```python
from build123d import *

# Parameters (mm, degrees)
BOSS_EXTRUDE1_DEPTH = 20
FILLET1_R           = 1
FILLET2_R           = 0.5


with BuildPart() as part:
    # Sketch1 → Boss-Extrude1 (new body)
    with BuildSketch(Plane(origin=(0, 0, 0), x_dir=(1, 0, 0), z_dir=(0, 1, 0))):
        Polygon((-2.4, 4.581818182), (2.4, 4.581818182), (7, 0.381818182), (2.4, 0.381818182), (2.4, -1.618181818), (10, -1.618181818), (10, -4.618181818), (-10, -4.618181818), (-10, -1.618181818), (-2.4, -1.618181818), (-2.4, 0.381818182), (-7, 0.381818182), align=None)
    extrude(amount=BOSS_EXTRUDE1_DEPTH)

    # Fillet1
    fillet1_edges = [part.edges().sort_by_distance(p)[0] for p in [
        (7, 10, -0.381818182),
        (-7, 10, -0.381818182),
        (-2.4, 10, -4.581818182),
        (2.4, 10, -4.581818182),
    ]]
    fillet(fillet1_edges, radius=FILLET1_R)

    # Fillet2
    fillet2_edges = [part.edges().sort_by_distance(p)[0] for p in [
        (2.4, 10, -0.381818182),
        (2.4, 10, 1.618181818),
        (-2.4, 10, 1.618181818),
        (-2.4, 10, -0.381818182),
    ]]
    fillet(fillet2_edges, radius=FILLET2_R)


solid = part.part
```
Here's how the part is built. I have some questions about the finished solid (model axes, mm). A direction names the side the tool comes from. Coordinates: 2 decimals unless noted, no trailing zeros. Order: outer loops, then holes, each group sorted by start corner. A loop starts at its lowest first (then second) coordinate and runs counter-clockwise, first axis right, second up. Notation, with made-up numbers: (2, 9) - (58, 9) arc R10 ccw to (58, 23) - close; hole circle Ø11 at (-18.5, -28.5). An arc over 180 degrees is marked (long way). One line per question, with ' | ' between items. Start each with the question number.
1. Please list where these lines run through material, in increasing order: line 1 along Z through (x, y) = (-4.25, 17.25); line 2 along Z through (x, y) = (4.5, 12.75); line 3 along Z through (x, y) = (-7, 19.25). Write a range as [from, to].
2. If we section it at C-C (x = 8): Write out the boundary of the cut face in (y, z), and give its area (3 significant figures).
3. If we section it at D-D (z = 0.75): Write out the boundary of the cut face in (x, y), and give its area (3 significant figures).
4. If we section it at A-A (y = 6.75): Write out the boundary of the cut face in (x, z).
5. I'm going to push flat-ended pins straight in: pin 1 Ø2 at (x, y) = (6, 12.5) entering from -Z; pin 2 Ø3.5 at (x, y) = (-7, 12.5) entering from -Z; pin 3 Ø1.5 at (x, y) = (-4, 13.5) entering from -Z; pin 4 Ø4 at (x, y) = (3.5, 2) entering from -Z. Where does each tip first touch, or does it pass through?
6. If we section it at B-B (x = 3.75): Write out the boundary of the cut face in (y, z).
7. Which directions (+Z, -Z, +X, -X, +Y, -Y) give clear straight access to the entire face, cutting with the end or side of a thin tool? Please do faces 4 (the flat face through (0, 10, -4.582)), 5 (the flat face through (-4, 10, -0.382)), 6 (the flat face through (6, 10, 1.618)).
8. If we mould it in two halves opening along Z, with no side actions, what happens to faces 1 (the flat face through (0, 0, 1)), 2 (the flat face through (0, 10, 4.618)), 3 (the flat face through (-2.4, 9.9, 0.6))? For each: released by +Z, released by -Z, zero draft, split by the parting line, or undercut.
Model answer:
1) line 1: z = [-2.89, -0.38], [1.62, 4.62] | line 2: z = [-2.66, -0.38], [1.62, 4.62] | line 3: z = [1.62, 4.62]
2) outline: (0, 1.62) - (20, 1.62) - (20, 4.62) - (0, 4.62) - close | area: 60.0 mm²
3) outline: (-2.4, 0) - (2.4, 0) - (2.4, 20) - (-2.4, 20) - close | area: 96.0 mm²
4) outline: (-10, 1.62) - (-2.9, 1.62) arc R0.5 cw to (-2.4, 1.12) - (-2.4, 0.12) arc R0.5 cw to (-2.9, -0.38) - (-4.42, -0.38) arc R1 ccw to (-5.1, -2.12) - (-2.69, -4.32) arc R1 ccw to (-2.01, -4.58) - (2.01, -4.58) arc R1 ccw to (2.69, -4.32) - (5.1, -2.12) arc R1 ccw to (4.42, -0.38) - (2.9, -0.38) arc R0.5 cw to (2.4, 0.12) - (2.4, 1.12) arc R0.5 cw to (2.9, 1.62) - (10, 1.62) - (10, 4.62) - (-10, 4.62) - close
5) pin 1: stops at z = -2.21 | pin 2: stops at z = -1.94 | pin 3: stops at z = -3.81 | pin 4: stops at z = -4.58
6) outline: (0, -3.35) - (20, -3.35) - (20, -0.38) - (0, -0.38) - close; (0, 1.62) - (20, 1.62) - (20, 4.62) - (0, 4.62) - close
7) face 4: -Z, +X, -X, +Y, -Y | face 5: -X, +Y, -Y | face 6: +X, +Y, -Y
8) face 1: zero draft | face 2: released by +Z | face 3: undercut
